The model under review builds one solid part; all positions refer to its coordinate system, in mm. Face numbers are marked on the shaded views. Coordinates: 2 decimals unless noted, no trailing zeros. Loops run counter-clockwise (first coordinate to the right, second up) from the corner with the lowest first, then second, coordinate; pieces in that order, holes last. Notation, with made-up numbers: M -37,80.25 L -27,80.25 A26 ccw -27,111.25 Z; hole C 45.25,-2.5 d11. An arc over 180 degrees is marked long. One line per item, written item: value.
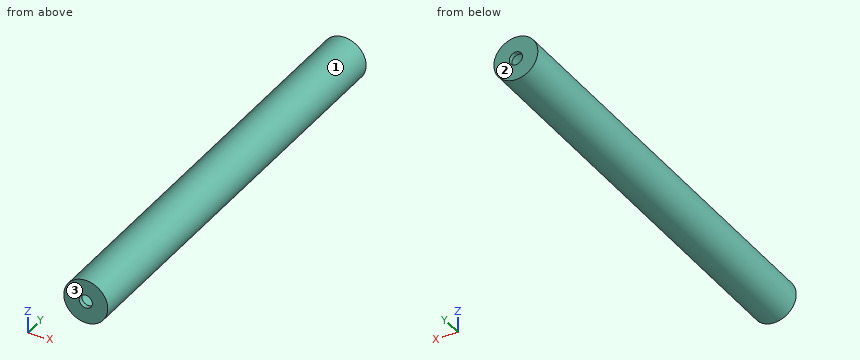
```python
from build123d import *

# Parameters (mm, degrees)
SKETCH1_R               = 10
BOSS_EXTRUDE1_DEPTH     = 200
SHELL1_T                = 2
SKETCH2_R               = 3
CUT_EXTRUDE1_DEPTH      = 1
CUT_EXTRUDE1_DEPTH_BACK = 201


with BuildPart() as part:
    # Sketch1 → Boss-Extrude1 (new body)
    with BuildSketch(Plane(origin=(0, 0, 0), x_dir=(1, 0, 0), z_dir=(0, 1, 0))):
        Circle(SKETCH1_R)
    extrude(amount=BOSS_EXTRUDE1_DEPTH)

    # Shell1 (no face opened: a closed hollow body)
    add(offset(amount=-SHELL1_T, mode=Mode.PRIVATE), mode=Mode.SUBTRACT)

    # Sketch2 → Cut-Extrude1 (cut, two sides)
    with BuildSketch(Plane(origin=(0, 200, 0), x_dir=(1, 0, 0), z_dir=(0, 1, 0))) as cut_extrude1_sk:
        Circle(SKETCH2_R)
    extrude(amount=CUT_EXTRUDE1_DEPTH, mode=Mode.SUBTRACT)
    extrude(cut_extrude1_sk.sketch, amount=-CUT_EXTRUDE1_DEPTH_BACK, mode=Mode.SUBTRACT)


solid = part.part
```
(1) Add section B-B on z = 0. State the section outline as (x, y) points, then the cut area to 3 significant figures.
Checks:
outline: M -10,0 L -3,0 L -3,2 L -8,2 L -8,198 L -3,198 L -3,200 L -10,200 Z; M 3,0 L 10,0 L 10,200 L 3,200 L 3,198 L 8,198 L 8,2 L 3,2 Z
area: 840 mm^2
(2) Add section C-C on y = 183. State the section outline as (x, z) points, then the cut area to 3 significant figures.
Checks:
outline: C 0,0 d20; hole C 0,0 d16
area: 113 mm^2
(3) Draft analysis for pull direction Y (two halves, no side actions). For the marked faces 1, 2 and 3, state which applies: pulls with the +Y half, pulls with the -Y half, needs draft (parallel to the pull), parting line crosses it, or undercut.
Checks:
face 1: needs draft
face 2: pulls with the +Y half
face 3: pulls with the -Y half
(4) To check wall thickness, follow L1, parallel to Z at x = 0, y = 145.5; L2, parallel to Y at x = 0.25, z = -6; L3, parallel to X at y = 0.95, z = 0. State the ranges of each line that lie inside material, in increasing order. Write a range as [from, to].
Checks:
L1: [-10, -8], [8, 10]
L2: [0, 2], [198, 200]
L3: [-10, -3], [3, 10]
(5) Add section A-A on x = 0. State the section outline as (y, z) points, then the cut area to 3 significant figures.
Checks:
outline: M 0,-10 L 200,-10 L 200,-3 L 198,-3 L 198,-8 L 2,-8 L 2,-3 L 0,-3 Z; M 0,3 L 2,3 L 2,8 L 198,8 L 198,3 L 200,3 L 200,10 L 0,10 Z
area: 840 mm^2
(6) Insertion check: pin 1 Ø1.5 at (x, y) = (0.5, 130) entering from +Z; pin 2 Ø3 at (y, z) = (146, -8) entering from -X; pin 3 Ø8 at (y, z) = (85.5, -4.5) entering from -X; pin 4 Ø1.5 at (y, z) = (56, -8) entering from +X. Each pin has a flat end and moves straight along its axis. Give the tip position at first contact, or say it passes through.
Checks:
pin 1: z = 10
pin 2: x = -7.6
pin 3: x = -9.99
pin 4: x = 6.89
